```python
from build123d import *

# Parameters (mm, degrees)
SKETCH1_W               = 254
SKETCH1_H               = 254
BASE_EXTRUDE_DEPTH      = 25.5
FILLET4_R               = 0.79375
FILLET4_OF_MIRROR3_R    = 0.79375
SKETCH4_R               = 6.35
CUT_EXTRUDE1_DEPTH      = 187.705650691
MIRROR2_COPY_1_SKETCH_R = 6.35
MIRROR2_COPY_1_DEPTH    = 187.705650691
SKETCH5_R               = 101.85
SKETCH5_R_2             = 101.6
CUT_EXTRUDE2_DEPTH      = 3.175
SKETCH7_R               = 101.6
CUT_EXTRUDE3_DEPTH      = 187.705650691


with BuildPart() as part:
    # Sketch1 → Base-Extrude (new, symmetric)
    with BuildSketch(Plane.XY):
        Rectangle(SKETCH1_W, SKETCH1_H)
    extrude(amount=BASE_EXTRUDE_DEPTH, both=True)

    # Cut-Sweep1: sweep along a path in Sketch3
    with BuildLine(Plane.XY) as cut_sweep1_path:
        Line((127, 127), (-127, 127))
    # Sketch2 → Cut-Sweep1 (sweep, cut)
    with BuildSketch(Plane(origin=(127, 0, 0), x_dir=(0, 0, -1), z_dir=(1, 0, 0))):
        with BuildLine():
            Line((-7.9375, 127), (7.9375, 127))
            Line((7.9375, 127), (9.590397866, 123.612719875))
            ThreePointArc((9.590397866, 123.612719875), (9.542015805, 122.686966067), (8.73125, 122.2375))
            Line((8.73125, 122.2375), (-8.73125, 122.2375))
            ThreePointArc((-8.73125, 122.2375), (-9.542015805, 122.686966067), (-9.590397866, 123.612719875))
            Line((-9.590397866, 123.612719875), (-7.9375, 127))
        make_face()
    cut_sweep1 = sweep(path=cut_sweep1_path.line, mode=Mode.SUBTRACT)

    # Fillet4
    fillet4_edges = [part.edges().sort_by_distance(p)[0] for p in [
        (0, 127, 7.9375),
        (0, 127, -7.9375),
    ]]
    fillet(fillet4_edges, radius=FILLET4_R)

    # Mirror3: Cut-Sweep1 across plane
    add(cut_sweep1.mirror(Plane.ZX), mode=Mode.SUBTRACT)

    # Fillet4 of Mirror3
    fillet4_of_mirror3_edges = [part.edges().sort_by_distance(p)[0] for p in [
        (0, -127, 7.9375),
        (0, -127, -7.9375),
    ]]
    fillet(fillet4_of_mirror3_edges, radius=FILLET4_OF_MIRROR3_R)

    # Sketch4 → Cut-Extrude1 (cut, through all)
    with BuildSketch(Plane.XY.offset(25.5)):
        with Locations((-101.6, 101.6)):
            Circle(SKETCH4_R)
    cut_extrude1 = extrude(amount=-CUT_EXTRUDE1_DEPTH, mode=Mode.SUBTRACT)

    # Mirror1: Cut-Extrude1 across plane
    add(cut_extrude1.mirror(Plane.ZX), mode=Mode.SUBTRACT)

    # Mirror2: Cut-Extrude1 across plane
    add(cut_extrude1.mirror(Plane(origin=(0, 0, 0), x_dir=(0, 0, 1), z_dir=(1, 0, 0))), mode=Mode.SUBTRACT)

    # Mirror2 copy 1 sketch → Mirror2 copy 1 (cut, through all)
    with BuildSketch(Plane(origin=(0, 0, 25.5), x_dir=(-1, 0, 0), z_dir=(0, 0, 1))):
        with Locations((-101.6, 101.6)):
            Circle(MIRROR2_COPY_1_SKETCH_R)
    extrude(amount=-MIRROR2_COPY_1_DEPTH, mode=Mode.SUBTRACT)

    # Sketch5 → Cut-Extrude2 (cut)
    with BuildSketch(Plane(origin=(0, 0, -25.5), x_dir=(-1, 0, 0), z_dir=(0, 0, -1))):
        Circle(SKETCH5_R)
        Circle(SKETCH5_R_2, mode=Mode.SUBTRACT)
    extrude(amount=-CUT_EXTRUDE2_DEPTH, mode=Mode.SUBTRACT)

    # Sketch7 → Cut-Extrude3 (cut, through all)
    with BuildSketch(Plane(origin=(0, 0, -25.5), x_dir=(-1, 0, 0), z_dir=(0, 0, -1))):
        Circle(SKETCH7_R)
    extrude(amount=-CUT_EXTRUDE3_DEPTH, mode=Mode.SUBTRACT)


solid = part.part
```
Here's how the part is built. I have some questions about the finished solid (model axes, mm). A direction names the side the tool comes from. Round coordinates to 2 decimals unless told otherwise and drop trailing zeros. Write each loop counter-clockwise with the first axis right and the second up, starting at its lowest first coordinate (ties: lowest second). Pieces come first, ordered by that corner, then holes. Notation, with made-up numbers: M -40,-28.75 L -31,-28.75 A25 ccw -31,-2.75 Z; hole C -38,0.25 d6. An arc over 180 degrees is marked long. Answer as CSV lines item,"result". Start each with the question number.
1. I need wall thicknesses on probe 1 along Y at (x, z) = (-1, 0.5); probe 2 along Y at (x, z) = (35, 13.5); probe 3 along Z at (x, y) = (61, -81.5) (3 decimals). Which ranges of each line are inside material? Lowest first, please.
2. Thinking about a two-plate mould opening in Z: for faces 1 (the flat face through (-86, 58, 25.5)), 2 (the flat face through (-2, -122.238, 0)), 3 (the cylindrical face through (-102.4, -107.9, 0.4)), which applies, released by +Z, released by -Z, zero draft, split by the parting line, or undercut?
3. On a 3-axis mill with a long thin cutter (end or side, diameter ignored), from which of +Z, -Z, +X, -X, +Y, -Y can I reach the whole of each face in a straight line? I mean faces 4 (the cylindrical face through (102.4, 107.9, 0.4)), 5 (the cylindrical face through (22.079, -99.428, -23.935)). Say none if no direction works.
4. Suppose I cut it at B-B on y = 0. Write out the boundary of the cut face in (x, z) (3 decimals), then the cut area to 3 significant figures.
5. Suppose I cut it at D-D on y = 85.5. Write out the boundary of the cut face in (x, z) (3 decimals), then the cut area to 3 significant figures.
6. Suppose I cut it at A-A on z = -15. Write out the boundary of the cut face in (x, y).
7. I'm going to push flat-ended pins straight in: pin 1 Ø1 at (x, z) = (-3, 0) entering from -Y; pin 2 Ø14.5 at (x, y) = (101.6, 101.6) entering from +Z; pin 3 Ø5 at (x, z) = (19.5, -3.5) entering from +Y. Where does each tip first touch, or does it pass through?
Check result:
1,probe 1,"y = -122.24 to -101.6, 101.6 to 122.24"
1,probe 2,"y = -127 to -95.38, 95.38 to 127"
1,probe 3,"z = -22.325 to 25.5"
2,face 1,"released by +Z"
2,face 2,"undercut"
2,face 3,"zero draft"
3,face 4,"+Z, -Z"
3,face 5,"-Z"
4,outline,"M -127,-25.5 L -101.85,-25.5 L -101.85,-22.325 L -101.6,-22.325 L -101.6,25.5 L -127,25.5 Z; M 101.6,-22.325 L 101.85,-22.325 L 101.85,-25.5 L 127,-25.5 L 127,25.5 L 101.6,25.5 Z"
4,area,"2,590 mm2"
5,outline,"M -127,-25.5 L -55.346,-25.5 L -55.346,-22.325 L -54.885,-22.325 L -54.885,25.5 L -127,25.5 Z; M 54.885,-22.325 L 55.346,-22.325 L 55.346,-25.5 L 127,-25.5 L 127,25.5 L 54.885,25.5 Z"
5,area,"7,350 mm2"
6,outline,"M -127,-127 L 127,-127 L 127,127 L -127,127 Z; hole C -101.6,-101.6 d12.7; hole C -101.6,101.6 d12.7; hole C 0,0 d203.2; hole C 101.6,-101.6 d12.7; hole C 101.6,101.6 d12.7"
7,pin 1,"stops at y = -122.24"
7,pin 2,"stops at z = 25.5"
7,pin 3,"stops at y = 122.24"
